Build history of the part. All positions in model axes, mm. A direction names the side the tool comes from. Give positions to 0.01 mm unless a question says otherwise; leave off trailing zeros. Loops run counter-clockwise (first coordinate to the right, second up) from the corner with the lowest first, then second, coordinate; pieces in that order, holes last. Notation, with made-up numbers: (46.25, 37.5) -> (92.25, 37.5) arc R17 ccw to (92.25, 44.5) -> close; hole circle Ø8 at (8.25, 21.5). An arc over 180 degrees is marked (long way). Answer as a JSON object with one key per item and string values. Group by question number.
from build123d import *

# Parameters (mm, degrees)
CROQUIS1_W              = 120
CROQUIS1_H              = 50.8
SALIENTE_EXTRUIR1_DEPTH = 12.7
CROQUIS2_W              = 12.7
CROQUIS2_H              = 50.8
SALIENTE_EXTRUIR2_DEPTH = 90
CROQUIS3_W              = 12.7
CROQUIS3_H              = 50.8
SALIENTE_EXTRUIR3_DEPTH = 90
CROQUIS4_W              = 140
CROQUIS4_H              = 50.8
SALIENTE_EXTRUIR4_DEPTH = 12.7
CROQUIS5_W              = 50.8
CROQUIS5_H              = 11.980562802
CROQUIS5_H_2            = 11.193759738
SALIENTE_EXTRUIR5_DEPTH = 13.65
CROQUIS6_W              = 12.7
CROQUIS6_H              = 50.8
SALIENTE_EXTRUIR6_DEPTH = 80


with BuildPart() as part:
    # Croquis1 → Saliente-Extruir1 (new body)
    with BuildSketch(Plane.XY):
        Rectangle(CROQUIS1_W, CROQUIS1_H)
    extrude(amount=SALIENTE_EXTRUIR1_DEPTH)

    # Croquis2 → Saliente-Extruir2 (add)
    with BuildSketch(Plane.XY.offset(12.7)):
        Rectangle(CROQUIS2_W, CROQUIS2_H)
    extrude(amount=SALIENTE_EXTRUIR2_DEPTH)

    # Croquis3 → Saliente-Extruir3 (add)
    with BuildSketch(Plane.XZ.offset(25.4)):
        with Locations((0, 77.3)):
            Rectangle(CROQUIS3_W, CROQUIS3_H)
    extrude(amount=SALIENTE_EXTRUIR3_DEPTH)

    # Croquis4 → Saliente-Extruir4 (add)
    with BuildSketch(Plane.ZY.offset(6.35)):
        with Locations((121.9, -90)):
            Rectangle(CROQUIS4_W, CROQUIS4_H)
    extrude(amount=SALIENTE_EXTRUIR4_DEPTH)

    # Croquis5 → Saliente-Extruir5 (add)
    with BuildSketch(Plane.ZY.offset(19.05)):
        with Locations((166.5, -109.409718599)):
            Rectangle(CROQUIS5_W, CROQUIS5_H)
        with Locations((166.5, -70.196879869)):
            Rectangle(CROQUIS5_W, CROQUIS5_H_2)
    extrude(amount=SALIENTE_EXTRUIR5_DEPTH)

    # Croquis6 → Saliente-Extruir6 (add)
    with BuildSketch(Plane(origin=(0, 25.4, 0), x_dir=(1, 0, 0), z_dir=(0, 1, 0))):
        with Locations((0, -77.3)):
            Rectangle(CROQUIS6_W, CROQUIS6_H)
    extrude(amount=SALIENTE_EXTRUIR6_DEPTH)


solid = part.part
(1) 3-axis set-ups, long thin cutter, end or side, ignore diameter. For faces 1 (the flat face through (-34, 0, 12.7)), 2 (the flat face through (0, -7, 102.7)), 3 (the flat face through (-26, -109, 141.1)): which of +Z, -Z, +X, -X, +Y, -Y reach the whole face in a straight line?
(2) Saw through at A-A on x = -25.5. List the corners of the cut face in (y, z).
(3) Probe line 1 along Z through (x, y) = (-20, -16); line 2 along X through (y, z) = (62, 91); line 3 along X through (y, z) = (-70, 170.5). List the from-to ranges inside material, lowest first. Write a range as [from, to].
(4) Pull direction Y, two halves, no side cores. Call faces 4 (the flat face through (-6.35, -90, 147)), 5 (the flat face through (-26, -103.419, 166)), 6 (the flat face through (-16, -64.6, 136)): pulls with the +Y half, pulls with the -Y half, needs draft (parallel to the pull), parting line crosses it, or undercut.
(5) Saw through at D-D on y = -19.5. List the corners of the cut face in (x, z), plus the area to 3 significant figures.
(6) Pin check, flat tips, straight feed: pin 1 (12 mm diameter, centred on x = 41, y = -10, fed in from -Z); pin 2 (7.5 mm diameter, centred on x = -10.5, y = -53.5, fed in from -Z); pin 3 (9 mm diameter, centred on y = -71.5, z = 158.5, fed in from -X); pin 4 (6 mm diameter, centred on x = 35.5, y = 5.5, fed in from +Z). Stop position of each tip, or through.
(7) Saw through at B-B on z = 152.5. List the corners of the cut face in (x, y).
(8) Saw through at C-C on x = -11. List the corners of the cut face in (y, z), plus the area to 3 significant figures.
Calculated:
{
 "1": {"face 1": "+Z, -X, +Y, -Y", "face 2": "+Z, +X, +Y, -Y", "face 3": "-Z, -X, +Y, -Y"},
 "2": {"outline": "(-115.4, 141.1) -> (-103.42, 141.1) -> (-103.42, 191.9) -> (-115.4, 191.9) -> close; (-75.79, 141.1) -> (-64.6, 141.1) -> (-64.6, 191.9) -> (-75.79, 191.9) -> close; (-25.4, 0) -> (25.4, 0) -> (25.4, 12.7) -> (-25.4, 12.7) -> close"},
 "3": {"line 1": "z = [0, 12.7]", "line 2": "x = [-6.35, 6.35]", "line 3": "x = [-32.7, -6.35]"},
 "4": {"face 4": "needs draft", "face 5": "undercut", "face 6": "pulls with the +Y half"},
 "5": {"outline": "(-60, 0) -> (60, 0) -> (60, 12.7) -> (6.35, 12.7) -> (6.35, 102.7) -> (-6.35, 102.7) -> (-6.35, 12.7) -> (-60, 12.7) -> close", "area": "2,670 mm^2"},
 "6": {"pin 1": "stops at z = 0", "pin 2": "passes through", "pin 3": "stops at x = -32.7", "pin 4": "stops at z = 12.7"},
 "7": {"outline": "(-32.7, -115.4) -> (-6.35, -115.4) -> (-6.35, -64.6) -> (-32.7, -64.6) -> (-32.7, -75.79) -> (-19.05, -75.79) -> (-19.05, -103.42) -> (-32.7, -103.42) -> close"},
 "8": {"outline": "(-115.4, 51.9) -> (-64.6, 51.9) -> (-64.6, 191.9) -> (-115.4, 191.9) -> close; (-25.4, 0) -> (25.4, 0) -> (25.4, 12.7) -> (-25.4, 12.7) -> close", "area": "7,760 mm^2"}
}
